Model file for the job. Use its own axes, mm. A direction names the side the tool comes from. Give positions to 0.01 mm unless a question says otherwise; leave off trailing zeros. Write each loop counter-clockwise with the first axis right and the second up, starting at its lowest first coordinate (ties: lowest second). Pieces come first, ordered by that corner, then holes. Notation, with made-up numbers: (-36.75, 86.25) - (12.25, 86.25) arc R17 ccw to (12.25, 92.25) - close; hole circle Ø3 at (-36.75, 47). An arc over 180 degrees is marked (long way). Use a Markdown table: item, result. Add a question column.
```python
from build123d import *

# Parameters (mm, degrees)
SKETCH1_W           = 72
SKETCH1_H           = 22
BOSS_EXTRUDE1_DEPTH = 20
SKETCH2_W           = 68
SKETCH2_H           = 18
CUT_EXTRUDE1_DEPTH  = 18
CUT_EXTRUDE2_DEPTH  = 30
SKETCH5_R           = 8.5
BOSS_EXTRUDE3_DEPTH = 67


with BuildPart() as part:
    # Sketch1 → Boss-Extrude1 (new body)
    with BuildSketch(Plane(origin=(0, 0, 0), x_dir=(1, 0, 0), z_dir=(0, 1, 0))):
        with Locations((-12.388663968, 12.75708502)):
            Rectangle(SKETCH1_W, SKETCH1_H)
    extrude(amount=BOSS_EXTRUDE1_DEPTH)

    # Sketch2 → Cut-Extrude1 (cut)
    with BuildSketch(Plane(origin=(0, 20, 0), x_dir=(1, 0, 0), z_dir=(0, 1, 0))):
        with Locations((-12.388663968, 12.75708502)):
            Rectangle(SKETCH2_W, SKETCH2_H)
    extrude(amount=-CUT_EXTRUDE1_DEPTH, mode=Mode.SUBTRACT)

    # Sketch4 → Cut-Extrude2 (cut)
    with BuildSketch(Plane.XY.offset(-1.75708502)):
        with BuildLine():
            Line((-46.388663968, 20), (-46.388663968, 14.00702655))
            Line((-46.388663968, 14.00702655), (-42.387974224, 14.00702655))
            Line((-42.387974224, 14.00702655), (-42.387974224, 17.5))
            ThreePointArc((-42.387974224, 17.5), (-41.655741177, 19.267766953), (-39.887974224, 20))
            Line((-39.887974224, 20), (-46.388663968, 20))
        make_face()
        with BuildLine():
            Line((0.111336032, 20), (-24.887974224, 20))
            ThreePointArc((-24.887974224, 20), (-23.120694993, 19.267968974), (-22.388663968, 17.500689744))
            Line((-22.388663968, 17.500689744), (-22.388663968, 13.429648774))
            Line((-22.388663968, 13.429648774), (-2.388663968, 13.429648774))
            Line((-2.388663968, 13.429648774), (-2.388663968, 17.5))
            ThreePointArc((-2.388663968, 17.5), (-1.656430921, 19.267766953), (0.111336032, 20))
        make_face()
        with BuildLine():
            Line((21.611336032, 20), (15.111336032, 20))
            ThreePointArc((15.111336032, 20), (16.879102985, 19.267766953), (17.611336032, 17.5))
            Line((17.611336032, 17.5), (17.611336032, 13.424239873))
            Line((17.611336032, 13.424239873), (21.611336032, 13.424239873))
            Line((21.611336032, 13.424239873), (21.611336032, 20))
        make_face()
    extrude(amount=-CUT_EXTRUDE2_DEPTH, mode=Mode.SUBTRACT)

    # Sketch5 → Boss-Extrude3 (add)
    with BuildSketch(Plane.ZY.offset(-21.611336032)):
        with Locations((-12.859898676, 12)):
            Circle(SKETCH5_R)
    extrude(amount=BOSS_EXTRUDE3_DEPTH)


solid = part.part
```
(1) Which spindle directions (+Z, -Z, +X, -X, +Y, -Y) get a long thin tool onto all of the face, cutting with end or side? Do faces 4 (the flat face through (-47, 20, -13)), 5 (the flat face through (-46.389, 11, -13)), 6 (the flat face through (-42.388, 16, -23)). Say none if no direction does.
(2) Band-saw the part on B-B (y = 12). Write the cut outline in (x, z), then the cut area to 3 significant figures.
(3) Band-saw the part on A-A (x = 13). Write the cut outline in (y, z), then the cut area to 3 significant figures.
(4) Band-saw the part on C-C (z = -3). Write the cut outline in (x, y).
(5) Flat gauge pins, fed straight in: pin 1 (1.6 mm diameter, centred on x = 20.5, z = -23, fed in from +Y); pin 2 (0.6 mm diameter, centred on x = -36, z = -2.5, fed in from +Y); pin 3 (2 mm diameter, centred on x = -45, z = -23, fed in from +Y); pin 4 (1.5 mm diameter, centred on x = -19.5, z = -10.5, fed in from -Y). Where does each tip first touch, or does it go through?
(6) Two-plate mould, pull along Z, no slides. Class faces 1 (the cylindrical face through (-41.675, 19.248, -2.743)), 2 (the flat face through (-13, 8, -1.757)), 3 (the flat face through (-45.389, 12, -13)): +Z half, -Z half, draft (parallel to the pull), parting line (faces both ways), or undercut.
(7) Band-saw the part on D-D (y = 5.5). Write the cut outline in (x, z).
(8) Probe probe 1 along Z at (x, y) = (1, 12); probe 2 along X at (y, z) = (3.25, -8.5); probe 3 along X at (y, z) = (11.75, -18). List the from-to ranges inside material, lowest first. Write a range as [from, to].
Model answer:
| question | item | result |
|---|---|---|
| 1 | face 4 | +Z, -Z, -X, +Y |
| 1 | face 5 | +Y |
| 1 | face 6 | -Z, +Y |
| 2 | outline | (-48.39, -23.76) - (23.61, -23.76) - (23.61, -1.76) - (-48.39, -1.76) - close; hole (-46.39, -21.76) - (21.61, -21.76) - (21.61, -21.36) - (-45.39, -21.36) - (-45.39, -4.36) - (21.61, -4.36) - (21.61, -3.76) - (-46.39, -3.76) - close |
| 2 | area | 1,500 mm^2 |
| 3 | outline | (0, -23.76) - (20, -23.76) - (20, -21.76) - (2, -21.76) - (2, -3.76) - (20, -3.76) - (20, -1.76) - (0, -1.76) - close; circle Ø17 at (12, -12.86) |
| 3 | area | 343 mm^2 |
| 4 | outline | (-48.39, 0) - (23.61, 0) - (23.61, 20) - (21.61, 20) - (21.61, 13.42) - (17.61, 13.42) - (17.61, 17.5) arc R2.5 ccw to (15.11, 20) - (0.11, 20) arc R2.5 ccw to (-2.39, 17.5) - (-2.39, 13.43) - (-22.39, 13.43) - (-22.39, 17.5) arc R2.5 ccw to (-24.89, 20) - (-39.89, 20) arc R2.5 ccw to (-42.39, 17.5) - (-42.39, 14.01) - (-46.39, 14.01) - (-46.39, 20) - (-48.39, 20) - close |
| 5 | pin 1 | stops at y = 13.42 |
| 5 | pin 2 | stops at y = 20 |
| 5 | pin 3 | stops at y = 14.01 |
| 5 | pin 4 | stops at y = 0 |
| 6 | face 1 | draft |
| 6 | face 2 | +Z half |
| 6 | face 3 | undercut |
| 7 | outline | (-48.39, -23.76) - (23.61, -23.76) - (23.61, -1.76) - (-48.39, -1.76) - close; hole (-46.39, -21.76) - (21.61, -21.76) - (21.61, -18.34) - (-45.39, -18.34) - (-45.39, -7.38) - (21.61, -7.38) - (21.61, -3.76) - (-46.39, -3.76) - close |
| 8 | probe 1 | z = [-23.76, -21.76], [-21.36, -4.36], [-3.76, -1.76] |
| 8 | probe 2 | x = [-48.39, -46.39], [21.61, 23.61] |
| 8 | probe 3 | x = [-48.39, -46.39], [-45.39, 23.61] |
